Verification items for the finished model (mm, model axes). Give positions to 0.01 mm unless a question says otherwise; leave off trailing zeros. Write each loop counter-clockwise with the first axis right and the second up, starting at its lowest first coordinate (ties: lowest second). Pieces come first, ordered by that corner, then holes. Notation, with made-up numbers: (70, 87) -> (114, 87) arc R8 ccw to (114, 94) -> close; hole circle Ø10 at (19.5, -5). An arc over 180 degrees is marked (long way). Use one line per item in the form item = value. Start each with the question number.
(1) Section check A-A, the plane y = 12. Record the cut outline in (x, z) (3 decimals).
(2) Section check B-B, the plane y = 41.5. Record the cut outline in (x, z) (3 decimals), plus the area to 3 significant figures.
(3) Release check for a two-part mould opening along X. For faces 1 (the face through (-0.69, 39.89, -3.1)), 2 (the face through (-0.69, 10.14, 3.1)), 3 (the face through (1.5, 30, -3)), 4 (the face through (-0.526, 21.576, -0.166)) record: pulls with the +X half, pulls with the -X half, needs draft (parallel to the pull), parting line crosses it, or undercut.
(4) Scan lines: L1, parallel to Z at x = 0, y = 8.75 (3 decimals); L2, parallel to Y at x = -2.5, z = -4.75; L3, parallel to X at y = 30.5, z = -0.25. Record each from-to range of solid material in increasing order.
(5) Depth check by flat-ended pin: pin 1 Ø8 at (x, y) = (-5.5, 15) entering from -Z; pin 2 Ø3 at (x, y) = (6, 26) entering from -Z; pin 3 Ø6 at (x, z) = (1.5, -6.5) entering from +Y. Enter the tip coordinate at first touch or a pass-through.
from build123d import *

# Parameters (mm, degrees)
CHANFREIN1_SIZE                     = 1
CHANFREIN2_SIZE                     = 0.5
DIAM_TRE_DU_PER_AGE_6_3_6_3_1_D     = 6.35
DIAM_TRE_DU_PER_AGE_6_3_6_3_1_DEPTH = 20
DIAM_TRE_DU_PER_AGE_6_3_6_3_1_TIP   = 1.907732465


with BuildPart() as part:
    # Esquisse1 → Révolution1 (revolve)
    with BuildSketch(Plane.XY):
        Polygon((0, 0), (8, 0), (8, 30), (3.175, 30), (3.175, 50), (0, 50), align=None)
    revolve(axis=Axis((0, 50, 0), (0, -1, 0)))

    # Chanfrein1
    chanfrein1_edges = [part.edges().sort_by_distance(p)[0] for p in [
        (-8, 30, 0),
    ]]
    chamfer(chanfrein1_edges, length=CHANFREIN1_SIZE)

    # Chanfrein2
    chanfrein2_edges = [part.edges().sort_by_distance(p)[0] for p in [
        (-8, 0, 0),
        (-3.175, 50, 0),
    ]]
    chamfer(chanfrein2_edges, length=CHANFREIN2_SIZE)

    # Diamètre du perçage Ø6.3 (6.3)1
    with Locations(Plane(origin=(0, 0, 0), x_dir=(-1, 0, 0), z_dir=(0, -1, 0))):
        with Locations((0, 0)):
            Hole(DIAM_TRE_DU_PER_AGE_6_3_6_3_1_D / 2, depth=DIAM_TRE_DU_PER_AGE_6_3_6_3_1_DEPTH)
            with Locations((0, 0, -(DIAM_TRE_DU_PER_AGE_6_3_6_3_1_DEPTH + DIAM_TRE_DU_PER_AGE_6_3_6_3_1_TIP / 2))):  # 118° drill point
                Cone(0, DIAM_TRE_DU_PER_AGE_6_3_6_3_1_D / 2, DIAM_TRE_DU_PER_AGE_6_3_6_3_1_TIP, mode=Mode.SUBTRACT)


solid = part.part
Completed:
q1.outline = circle Ø16 at (0, 0); hole circle Ø6.35 at (0, 0)
q2.outline = circle Ø6.35 at (0, 0)
q2.area = 31.7 mm²
q3.face_1 = parting line crosses it
q3.face_2 = undercut
q3.face_3 = needs draft
q3.face_4 = undercut
q4.L1 = -8 to -3.175, 3.175 to 8
q4.L2 = 0 to 30
q4.L3 = -3.17 to 3.17
q5.pin_1 = -7.86
q5.pin_2 = -6.61
q5.pin_3 = 30
